Build history of the part. All positions in model axes, mm. A direction names the side the tool comes from. Coordinates: 2 decimals unless noted, no trailing zeros. Loops run counter-clockwise (first coordinate to the right, second up) from the corner with the lowest first, then second, coordinate; pieces in that order, holes last.
(1) Flat gauge pins, fed straight in: P1, Ø6, axis at y = 77.5, z = -3.5, coming from the -X side; P2, Ø2, axis at x = 4, y = 115, coming from the -Z side; P3, Ø5, axis at x = -3, y = 84.5, coming from the -Z side. Where does each tip first touch, or does it go through?
(2) Slice it at D-D (y = 10.5). Give the cut face in (x, z).
(3) Slice it at A-A (z = 0). Give the cut face in (x, y), and give its area (3 significant figures).
(4) Slice it at C-C (y = 34.5). Give the cut face in (x, z).
(5) Slice it at B-B (x = 0). Give the cut face in (y, z).
(6) Tool access for faces 1 (the face through (4, 18, 4)), 2 (the face through (1.802, 75.681, 5.723)), 3 (the face through (4, 135, -4)): list every direction of +Z, -Z, +X, -X, +Y, -Y with a clear straight run to the whole face (end or side of a thin tool).
(7) Wall check: L1, parallel to Z at x = -0.25, y = 50; L2, parallel to Y at x = 5, z = 2.5; L3, parallel to X at y = 117, z = 2. Give the ranges that are in metal, low to high.
from build123d import *

# Parameters (mm, degrees)
SKETCH_1_R          = 6
EXTRUDE_1_DEPTH     = 150
CUT_EXTRUDE_START   = -15
SKETCH_2_R          = 6
SKETCH_2_R_2        = 5
CUT_EXTRUDE_1_DEPTH = 15
SKETCH_3_R          = 6
SKETCH_3_R_2        = 5
CUT_EXTRUDE_2_DEPTH = 18


with BuildPart() as part:
    # ｽｹｯﾁ1 → ﾎﾞｽ - 押し出し1 (new body)
    with BuildSketch(Plane(origin=(0, 0, 0), x_dir=(1, 0, 0), z_dir=(0, 1, 0))):
        with Locations(Location((0, 0, 0), (0, 0, 270))):
            Circle(SKETCH_1_R)
    extrude(amount=EXTRUDE_1_DEPTH)

    # ｽｹｯﾁ2 → ｶｯﾄ - 押し出し1 (cut)
    with BuildSketch(Plane(origin=(0, 150, 0), x_dir=(1, 0, 0), z_dir=(0, 1, 0)).offset(CUT_EXTRUDE_START)):
        with Locations(Location((0, 0, 0), (0, 0, 270))):
            Circle(SKETCH_2_R)
        with Locations(Location((0, 0, 0), (0, 0, 270))):
            Circle(SKETCH_2_R_2, mode=Mode.SUBTRACT)
    extrude(amount=CUT_EXTRUDE_1_DEPTH, mode=Mode.SUBTRACT)

    # ｽｹｯﾁ3 → ｶｯﾄ - 押し出し2 (cut)
    with BuildSketch(Plane(origin=(0, 0, 0), x_dir=(-1, 0, 0), z_dir=(0, -1, 0))):
        with Locations(Location((0, 0, 0), (0, 0, 90))):
            Circle(SKETCH_3_R)
        with Locations(Location((0, 0, 0), (0, 0, 270))):
            Circle(SKETCH_3_R_2, mode=Mode.SUBTRACT)
    extrude(amount=-CUT_EXTRUDE_2_DEPTH, mode=Mode.SUBTRACT)


solid = part.part
Response values:
1. P1: stops at x = -5.98
1. P2: stops at z = -5.2
1. P3: stops at z = -5.98
2. outline: circle Ø10 at (0, 0)
3. outline: (-6, 18) - (-5, 18) - (-5, 0) - (5, 0) - (5, 18) - (6, 18) - (6, 135) - (5, 135) - (5, 150) - (-5, 150) - (-5, 135) - (-6, 135) - close
3. area: 1,730 mm2
4. outline: circle Ø12 at (0, 0)
5. outline: (0, -5) - (18, -5) - (18, -6) - (135, -6) - (135, -5) - (150, -5) - (150, 5) - (135, 5) - (135, 6) - (18, 6) - (18, 5) - (0, 5) - close
6. face 1: -Y
6. face 2: +Y, -Y
6. face 3: +Y
7. L1: z = -5.99 to 5.99
7. L2: y = 18 to 135
7. L3: x = -5.66 to 5.66
